Geometry: final body of the model. Coordinates: model frame, mm. Give positions to 0.01 mm unless a question says otherwise; leave off trailing zeros. Loops run counter-clockwise (first coordinate to the right, second up) from the corner with the lowest first, then second, coordinate; pieces in that order, holes last. Notation, with made-up numbers: (-38, 17) -> (12, 17) arc R30 cw to (12, 48) -> close; hole circle Ø1 at (5, -30.75). An arc over 180 degrees is marked (long way). Answer in a Markdown table with one row per item. Add a question column.
from build123d import *


with BuildPart() as part:
    # Bottle_Liner_Top Sketch → Bottle_Liner_Top (revolve)
    with BuildSketch(Plane.XY, mode=Mode.PRIVATE) as bottle_liner_top_sk:
        Polygon((3.175, 64.694892683), (2.38125, 65.493853894), (1.5875, 66.260295916), (0.79375, 66.99533651), (0, 67.7), (-0.79375, 68.375226954), (-1.5875, 69.021882544), (-2.38125, 69.640763827), (-3.175, 70.232606084), (-3.175, 74.4485), (3.175, 70.5115), align=None)
    revolve(bottle_liner_top_sk.sketch.rotate(Axis((-300, 0, 0), (1, 0, 0)), 90), axis=Axis((-300, 0, 0), (1, 0, 0)))


solid = part.part
(1) Pin query (flat end, axial travel): pin 1 Ø10 at (y, z) = (-37.5, 43.5) entering from +X; pin 2 Ø3 at (x, y) = (-0.5, -19.5) entering from -Z; pin 3 Ø1.5 at (x, y) = (0.5, 30.5) entering from -Z; pin 4 Ø1.5 at (x, y) = (1.5, -56) entering from +Z. Return the tip coordinate at first contact, or that it passes through.
(2) Material intervals for line 1 along Y through (x, z) = (-0.25, -23.5); line 2 along Z through (x, y) = (-1.75, -45); line 3 along Y through (x, z) = (-0.5, 22), sorted ascending. Write a range as from..to.
(3) Cut plane A-A on y = 0. Return the cut outline in (x, z) (1 decimal).
Answer list:
| question | item | result |
|---|---|---|
| 1 | pin 1 | passes through |
| 1 | pin 2 | stops at z = -71.18 |
| 1 | pin 3 | stops at z = -66.03 |
| 1 | pin 4 | stops at z = 45.72 |
| 2 | line 1 | y = -68.73..-63.72, 63.72..68.73 |
| 2 | line 2 | z = -58.2..-52.5, 52.5..58.2 |
| 2 | line 3 | y = -69.39..-64.48, 64.48..69.39 |
| 3 | outline | (-3.2, -74.4) -> (3.2, -70.5) -> (3.2, -64.7) -> (2.4, -65.5) -> (1.6, -66.3) -> (0.8, -67) -> (0, -67.7) -> (-0.8, -68.4) -> (-1.6, -69) -> (-2.4, -69.6) -> (-3.2, -70.2) -> close; (-3.2, 70.2) -> (-2.4, 69.6) -> (-1.6, 69) -> (-0.8, 68.4) -> (0, 67.7) -> (0.8, 67) -> (1.6, 66.3) -> (2.4, 65.5) -> (3.2, 64.7) -> (3.2, 70.5) -> (-3.2, 74.4) -> close |
